Input: part model. Units: mm. Frame: model coordinates. A direction names the side the tool comes from. Coordinates: 2 decimals unless noted, no trailing zeros. Loops run counter-clockwise (first coordinate to the right, second up) from the corner with the lowest first, then second, coordinate; pieces in that order, holes last.
(1) Section A-A, the plane x = 15. Return loops of the section in (y, z), then the cut area to 3 significant figures.
(2) Mould query, pull axis Y, two halves, no side actions, for faces 5 (the face through (16.1, -6, 0.8)), 6 (the face through (-13, -3, 2)), 7 (the face through (-17, 0, 1)), 8 (the face through (-15.238, 13.926, 0.811)). Classes: released by +Y, released by -Y, zero draft, split by the parting line, or undercut.
(3) Section D-D, the plane x = -15. Return loops of the section in (y, z).
(4) Line query: L1, parallel to Y at x = 15, z = 0.7; L2, parallel to X at y = -6, z = 0.9; L3, parallel to Z at x = -4, y = -13. Output: solid intervals per line, ascending.
(5) Section C-C, the plane y = -6. Return loops of the section in (x, z).
(6) Set-up query: faces 1 (the face through (-15.5, 0, 2)), 2 (the face through (-2.17, -9.76, 3.18)), 3 (the face through (-10.5, 0, 2)), 4 (the face through (-16.2, 17.3, 0.8)). Return all of +Z, -Z, +X, -X, +Y, -Y with unobstructed straight access to the full face (end or side cutting, diameter ignored); none if empty.
(7) Contact query for flat-ended pins moving along their axis: P1, Ø3.5, axis at x = 15, y = 6, coming from the +Z side; P2, Ø1.1, axis at y = -1, z = 2.5, coming from the -X side; P3, Ø1, axis at x = 4, z = 4, coming from the -Y side. Output: stop coordinate, or through.
(8) Section B-B, the plane y = 15. Return loops of the section in (x, z), then the cut area to 3 significant figures.
```python
from build123d import *

# Parameters (mm, degrees)
SKETCH1_W           = 34
SKETCH1_H           = 36
BOSS_EXTRUDE1_DEPTH = 1.6
CHAMFER1_SIZE       = 1.5
SKETCH2_R           = 1.1
CUT_EXTRUDE1_DEPTH  = 25.810481656
SKETCH3_R           = 10
BOSS_EXTRUDE2_DEPTH = 3.2
SKETCH4_W           = 5
SKETCH4_H           = 6
BOSS_EXTRUDE3_DEPTH = 1


with BuildPart() as part:
    # Sketch1 → Boss-Extrude1 (new body)
    with BuildSketch(Plane.XY):
        Rectangle(SKETCH1_W, SKETCH1_H)
    extrude(amount=BOSS_EXTRUDE1_DEPTH)

    # Chamfer1
    chamfer1_edges = [part.edges().sort_by_distance(p)[0] for p in [
        (-17, 18, 0.8),
        (17, 18, 0.8),
        (17, -18, 0.8),
        (-17, -18, 0.8),
    ]]
    chamfer(chamfer1_edges, length=CHAMFER1_SIZE)

    # Sketch2 → Cut-Extrude1 (cut, through all)
    with BuildSketch(Plane.XY.offset(1.6)):
        with Locations((-15, 15)):
            Circle(SKETCH2_R)
        with Locations((15, 6)):
            Circle(SKETCH2_R)
        with Locations(Location((-15, -15, 0), (0, 0, 180))):
            Circle(SKETCH2_R)
        with Locations((15, -15)):
            Circle(SKETCH2_R)
        with Locations(Location((15, 15, 0), (0, 0, 180))):
            Circle(SKETCH2_R)
        with Locations(Location((15, -6, 0), (0, 0, 180))):
            Circle(SKETCH2_R)
    extrude(amount=-CUT_EXTRUDE1_DEPTH, mode=Mode.SUBTRACT)

    # Sketch3 → Boss-Extrude2 (add)
    with BuildSketch(Plane.XY.offset(1.6)):
        Circle(SKETCH3_R)
    extrude(amount=BOSS_EXTRUDE2_DEPTH)

    # Sketch4 → Boss-Extrude3 (add)
    with BuildSketch(Plane.XY.offset(1.6)):
        with Locations((-13, 0)):
            Rectangle(SKETCH4_W, SKETCH4_H)
    extrude(amount=BOSS_EXTRUDE3_DEPTH)


solid = part.part
```
Report:
1. outline: (-18, 0) - (-16.1, 0) - (-16.1, 1.6) - (-18, 1.6) - close; (-13.9, 0) - (-7.1, 0) - (-7.1, 1.6) - (-13.9, 1.6) - close; (-4.9, 0) - (4.9, 0) - (4.9, 1.6) - (-4.9, 1.6) - close; (7.1, 0) - (13.9, 0) - (13.9, 1.6) - (7.1, 1.6) - close; (16.1, 0) - (18, 0) - (18, 1.6) - (16.1, 1.6) - close
1. area: 43.5 mm2
2. face 5: undercut
2. face 6: released by -Y
2. face 7: zero draft
2. face 8: undercut
3. outline: (-18, 0) - (-16.1, 0) - (-16.1, 1.6) - (-18, 1.6) - close; (-13.9, 0) - (13.9, 0) - (13.9, 1.6) - (3, 1.6) - (3, 2.6) - (-3, 2.6) - (-3, 1.6) - (-13.9, 1.6) - close; (16.1, 0) - (18, 0) - (18, 1.6) - (16.1, 1.6) - close
4. L1: y = -18 to -16.1, -13.9 to -7.1, -4.9 to 4.9, 7.1 to 13.9, 16.1 to 18
4. L2: x = -17 to 13.9, 16.1 to 17
4. L3: z = 0 to 1.6
5. outline: (-17, 0) - (13.9, 0) - (13.9, 1.6) - (8, 1.6) - (8, 4.8) - (-8, 4.8) - (-8, 1.6) - (-17, 1.6) - close; (16.1, 0) - (17, 0) - (17, 1.6) - (16.1, 1.6) - close
6. face 1: +Z, -X, +Y, -Y
6. face 2: +Z
6. face 3: +Z, +Y, -Y
6. face 4: +Z, -Z, -X, +Y
7. P1: stops at z = 1.6
7. P2: stops at x = -15.5
7. P3: stops at y = -9.37
8. outline: (-17, 0) - (-16.1, 0) - (-16.1, 1.6) - (-17, 1.6) - close; (-13.9, 0) - (13.9, 0) - (13.9, 1.6) - (-13.9, 1.6) - close; (16.1, 0) - (17, 0) - (17, 1.6) - (16.1, 1.6) - close
8. area: 47.4 mm2
